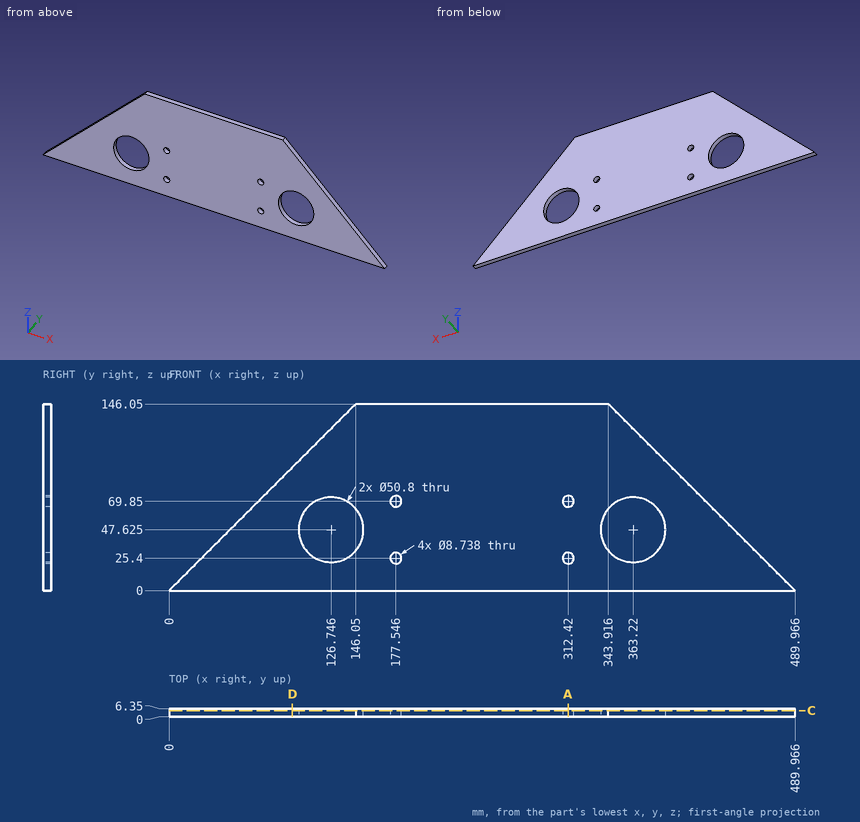
Geometry check sheet. Reference: drawing and pictorial views, mm from the part's lowest x, y, z. Round coordinates to 2 decimals unless told otherwise and drop trailing zeros. Order: outer loops, then holes, each group sorted by start corner. A loop starts at its lowest first (then second) coordinate and runs counter-clockwise, first axis right, second up. Notation, with made-up numbers: M 75.5,43 L 126.5,43 A10 cw 126.5,52 Z; hole C 37.25,-18.75 d10. An arc over 180 degrees is marked long. One line per item, written item: value. Start each with the question number.
1. Section check A-A on x = 312.42. Enter the section's corners in (y, z).
2. Section check C-C on y = 4.75. Give the number of separate pieces and of enclosed holes in the cut face, and give its area (3 significant figures).
3. Scan lines: line 1 along Z through (x, y) = (312.42, 4); line 2 along X through (y, z) = (4.75, 27) (1 decimal); line 3 along Z through (x, y) = (431, 2.25) (1 decimal). Record each from-to range of solid material in increasing order.
4. Section check D-D on x = 96.5. Enter the section's corners in (y, z), and give its area (3 significant figures).
5. Gauge pin test, flat ends, axial feed: P1, Ø14, axis at x = 177.546, z = 25.4, coming from the -Y side; P2, Ø3, axis at y = 0.5, z = 89.5, coming from the -X side; P3, Ø1.5, axis at y = 4, z = 96, coming from the +X side (1 decimal); P4, Ø1.5, axis at y = 3.5, z = 44.5, coming from the -X side. Record the tip position at first contact, or that the pin passes through.
Results found:
1. outline: M 0,0 L 6.35,0 L 6.35,21.03 L 0,21.03 Z; M 0,29.77 L 6.35,29.77 L 6.35,65.48 L 0,65.48 Z; M 0,74.22 L 6.35,74.22 L 6.35,146.05 L 0,146.05 Z
2. separate pieces: 1
2. enclosed holes: 6
2. area: 45,900 mm^2
3. line 1: 0 to 21.03, 29.77 to 65.48, 74.22 to 146.05
3. line 2: 27 to 111.9, 141.6 to 173.5, 181.6 to 308.4, 316.5 to 348.4, 378 to 463
3. line 3: 0 to 59
4. outline: M 0,0 L 6.35,0 L 6.35,96.5 L 0,96.5 Z
4. area: 613 mm^2
5. P1: y = 0
5. P2: x = 88
5. P3: x = 394.7
5. P4: x = 43.75
